CAD build for the part. Positions are in the model's coordinates, mm. A direction names the side the tool comes from. Coordinates: 2 decimals unless noted, no trailing zeros. Loops run counter-clockwise (first coordinate to the right, second up) from the corner with the lowest first, then second, coordinate; pieces in that order, holes last. Notation, with made-up numbers: (9.5, 33) -> (31.5, 33) arc R7 cw to (31.5, 40) -> close; hole circle Ø3 at (-7.75, 19.25). An arc over 180 degrees is marked (long way). Write each question's results on one line, items separated by ' | '.
Autodesk Inventor part; units mm, degrees
ref_plane "YZ Plane" through (0, 0, 0) normal (1, 0, 0) x (0, 1, 0)
ref_plane "XZ Plane" through (0, 0, 0) normal (0, 1, 0) x (-1, 0, 0)
ref_plane "XY Plane" through (0, 0, 0) normal (0, 0, 1) x (1, 0, 0)
sketch "Skizze1" plane through (0, 0, 0) normal (1, 0, 0) x (0, 1, 0)
  line L0 (5, 92.5) -> (0, 92.5)
  line L1 (0, 92.5) -> (0, 0)
  line L2 (0, 0) -> (5, 0)
  line L3 (5, 0) -> (5, 92.5)
  line L4 (-37, 0) -> (12, 0)
  line L5 (0, 0) -> (-30, 0)
  line L6 (-30, 0) -> (-30, 5)
  line L7 (-30, 5) -> (0, 5)
  line L8 (0, 5) -> (0, 0)
  dimension "d0" = 5
  dimension "d1" = 92.5
  dimension "d3" = 5
  dimension "d4" = 35
extrude "Extrusion1" add sketch "Skizze1" along normal mid plane 60
fillet "Rundung1" radius 2 1 edges at (0, 0, 5)
fillet "Rundung2" radius 7 1 edges at (0, 5, 0)
sketch "Skizze2" plane through (-30, 0, 92.5) normal (0, -1, 0) x (1, 0, 0)
  line L0 (0, -92.5) -> (60, -92.5)
  line L1 (60, 0) -> (60, -85.5)
  line L2 (0, -85.5) -> (0, 0)
  line L3 (10, -4) -> (10, -4)
  line L4 (12.25, -6.25) -> (12.25, -7.75)
  line L5 (10, -10) -> (10, -10)
  line L6 (7.75, -7.75) -> (7.75, -6.25)
  line L7 (7.75, -4) -> (12.25, -10) construction
  line L8 (12.25, -4) -> (7.75, -10) construction
  arc A0 (10, -4) -> (7.75, -6.25) centre (10, -6.25) ccw
  arc A1 (12.25, -6.25) -> (10, -4) centre (10, -6.25) ccw
  arc A2 (7.75, -7.75) -> (10, -10) centre (10, -7.75) ccw
  arc A3 (10, -10) -> (12.25, -7.75) centre (10, -7.75) ccw
  line L9 (60, 0) -> (0, 0)
  point P0 (30, -92.5)
  point P1 (10, -7)
  point P2 (10, -4)
  dimension "d12" = 60
  dimension "d13" = 10
  dimension "d14" = 4.5
  dimension "d15" = 6
  dimension "d16" = 2.25
  dimension "d39" = 7
extrude "Extrusion2" cut sketch "Skizze2" against normal blind 50
pattern_linear "Rechteckige Anordnung1" count 2 spacing 40 along (1, 0, 0) count 2 spacing 19 along (0, 0, -1) of "Extrusion2"
sketch "Skizze3" plane through (-30, -30, 5) normal (0, 0, 1) x (1, 0, 0)
  line L0 (7, 11) -> (7, 11)
  line L1 (10.3, 7.7) -> (10.3, 6.3)
  line L2 (7, 3) -> (7, 3)
  line L3 (3.7, 6.3) -> (3.7, 7.7)
  line L4 (3.7, 11) -> (10.3, 3) construction
  line L5 (10.3, 11) -> (3.7, 3) construction
  arc A0 (7, 11) -> (3.7, 7.7) centre (7, 7.7) ccw
  arc A1 (3.7, 6.3) -> (7, 3) centre (7, 6.3) ccw
  arc A2 (7, 3) -> (10.3, 6.3) centre (7, 6.3) ccw
  arc A3 (10.3, 7.7) -> (7, 11) centre (7, 7.7) ccw
  line L6 (0, 0) -> (0, 28)
  line L7 (0, 0) -> (60, 0)
  point P0 (30, 30)
  point P1 (7, 7)
  point P2 (7, 3)
  dimension "d26" = 6.6
  dimension "d27" = 8
  dimension "d28" = 3.3
  dimension "d29" = 7
  dimension "d30" = 7
extrude "Extrusion3" cut sketch "Skizze3" against normal through all
pattern_linear "Rechteckige Anordnung2" count 2 spacing 46 along (1, 0, 0) count 2 spacing 13 along (0, 1, 0) of "Extrusion3"
properties part number "TS_V1_Fallmagazin_Haltewinkel_Fuehrung_int"
1) Which spindle directions (+Z, -Z, +X, -X, +Y, -Y) get a long thin tool onto all of the face, cutting with end or side? Do faces 4 (the cylindrical face through (-23, -27, 3)), 5 (the flat face through (0, -16, 5)), 6 (the cylindrical face through (-20, 2.5, 82.5)), 7 (the flat face through (0, -30, 2)), 8 (the flat face through (0, 5, 49)). Say none if no direction does.
Outcome:
face 4: +Z, -Z | face 5: +Z, +X, -X, -Y | face 6: +Y, -Y | face 7: +Z, -Z, +X, -X, -Y | face 8: +Z, -Z, +X, -X, +Y
2) Pin check, flat tips, straight feed: pin 1 (1.5 mm diameter, centred on x = 21.5, y = -21.5, fed in from +Z); pin 2 (3 mm diameter, centred on x = -19, z = 21, fed in from -Y). Stop position of each tip, or through.
Outcome:
pin 1: passes through | pin 2: stops at y = 0
3) Two-plate mould, pull along X, no slides. Class faces 1 (the cylindrical face through (-0.4, 3, 2.1)), 2 (the cylindrical face through (23, -19, 3)), 3 (the flat face through (30, 0.4, 39.6)): pulls with the +X half, pulls with the -X half, needs draft (parallel to the pull), parting line crosses it, or undercut.
Outcome:
face 1: needs draft | face 2: undercut | face 3: pulls with the +X half
4) Slice it at A-A (x = -14). Write the cut outline in (y, z).
Outcome:
outline: (-30, 0) -> (-2, 0) arc R7 ccw to (5, 7) -> (5, 92.5) -> (0, 92.5) -> (0, 7) arc R2 cw to (-2, 5) -> (-30, 5) -> close
5) Drill centre lines: L1, parallel to Z at x = 8.5, y = -19; L2, parallel to Z at x = 11.5, y = -1. Where is each one in solid material? Low to high. Write a range as from..to.
Outcome:
L1: z = 0..5 | L2: z = 0.07..5.27
6) Slice it at B-B (y = 3.5). Write the cut outline in (x, z).
Outcome:
outline: (-30, 2.67) -> (30, 2.67) -> (30, 92.5) -> (-30, 92.5) -> close; hole (-22.25, 65.75) arc R2.25 ccw to (-17.75, 65.75) -> (-17.75, 67.25) arc R2.25 ccw to (-22.25, 67.25) -> close; hole (-22.25, 84.75) arc R2.25 ccw to (-17.75, 84.75) -> (-17.75, 86.25) arc R2.25 ccw to (-22.25, 86.25) -> close; hole (17.75, 65.75) arc R2.25 ccw to (22.25, 65.75) -> (22.25, 67.25) arc R2.25 ccw to (17.75, 67.25) -> close; hole (17.75, 84.75) arc R2.25 ccw to (22.25, 84.75) -> (22.25, 86.25) arc R2.25 ccw to (17.75, 86.25) -> close
7) Slice it at C-C (z = 25.5). Write the cut outline in (x, y), then the cut area to 3 significant figures.
Outcome:
outline: (-30, 0) -> (30, 0) -> (30, 5) -> (-30, 5) -> close | area: 300 mm^2
